```python
from build123d import *

# Parameters (mm, degrees)
BOSS_EXTRUDE1_DEPTH = 20
SKETCH2_W           = 700
SKETCH2_H           = 15
BOSS_EXTRUDE2_DEPTH = 20
SKETCH6_W           = 10
SKETCH6_H           = 10
BOSS_EXTRUDE3_DEPTH = 500
BOSS_EXTRUDE4_DEPTH = 5
SKETCH8_W           = 10
SKETCH8_H           = 10
BOSS_EXTRUDE5_DEPTH = 495
SKETCH4_W           = 700
SKETCH4_H           = 12.5
CUT_EXTRUDE2_DEPTH  = 5


with BuildPart() as part:
    # Sketch1 → Boss-Extrude1 (new body)
    with BuildSketch(Plane(origin=(0, 0, 0), x_dir=(1, 0, 0), z_dir=(0, 1, 0))):
        Polygon((0, 404.145188433), (-350, -202.072594216), (350, -202.072594216), align=None)
        Polygon((0, 381.051177665), (-330, -190.525588833), (330, -190.525588833), align=None, mode=Mode.SUBTRACT)
    extrude(amount=BOSS_EXTRUDE1_DEPTH)

    # Sketch2 → Boss-Extrude2 (add)
    with BuildSketch(Plane(origin=(0, 0, 0), x_dir=(1, 0, 0), z_dir=(0, 1, 0))):
        with Locations((0, -209.572594216)):
            Rectangle(SKETCH2_W, SKETCH2_H)
    extrude(amount=BOSS_EXTRUDE2_DEPTH)

    # Sketch6 → Boss-Extrude3 (add)
    with BuildSketch(Plane(origin=(0, 20, 0), x_dir=(1, 0, 0), z_dir=(0, 1, 0))):
        with Locations((40, -196.3)):
            Rectangle(SKETCH6_W, SKETCH6_H)
    extrude(amount=BOSS_EXTRUDE3_DEPTH)

    # Sketch7 → Boss-Extrude4 (add)
    with BuildSketch(Plane(origin=(0, 20, 0), x_dir=(1, 0, 0), z_dir=(0, 1, 0))):
        Polygon((62.94207364, 295.126318955), (-62.94207364, 295.126318955), (-95, 239.600361714), (95, 239.600361714), align=None)
    extrude(amount=BOSS_EXTRUDE4_DEPTH)

    # Sketch8 → Boss-Extrude5 (add)
    with BuildSketch(Plane(origin=(0, 25, 0), x_dir=(1, 0, 0), z_dir=(0, 1, 0))):
        with Locations((40, 250)):
            Rectangle(SKETCH8_W, SKETCH8_H)
    extrude(amount=BOSS_EXTRUDE5_DEPTH)

    # Sketch4 → Cut-Extrude2 (cut)
    with BuildSketch(Plane(origin=(0, 20, 0), x_dir=(1, 0, 0), z_dir=(0, 1, 0))):
        with Locations((0, -208.322594216)):
            Rectangle(SKETCH4_W, SKETCH4_H)
    extrude(amount=-CUT_EXTRUDE2_DEPTH, mode=Mode.SUBTRACT)


solid = part.part
```
The listing builds one solid part. Answer for the finished solid, in the listing's coordinates (mm). A direction names the side the tool comes from. Give positions to 0.01 mm unless a question says otherwise; leave off trailing zeros. Order: outer loops, then holes, each group sorted by start corner. A loop starts at its lowest first (then second) coordinate and runs counter-clockwise, first axis right, second up. Notation, with made-up numbers: (2.5, -6) -> (45.5, -6) arc R28 cw to (45.5, 22) -> close; hole circle Ø4 at (20, -4.75). An arc over 180 degrees is marked (long way). One line per item, written item: value.
1) Find section C-C, the plane x = 269. Determine the outline of the cut face in (y, z), plus the area to 3 significant figures.
Reported:
outline: (0, 61.78) -> (20, 61.78) -> (20, 84.87) -> (0, 84.87) -> close; (0, 190.53) -> (20, 190.53) -> (20, 202.07) -> (15, 202.07) -> (15, 214.57) -> (20, 214.57) -> (20, 217.07) -> (0, 217.07) -> close
area: 930 mm^2
2) A tool of negligible diameter and unlimited length cuts with its end or side. For faces 3 (the flat face through (-2, 0, 204)), 4 (the flat face through (-1, 20, -268)), from which of +Z, -Z, +X, -X, +Y, -Y can it reach the whole face along a straight path? Write none if from no direction.
Reported:
face 3: +Z, -Z, +X, -X, -Y
face 4: -Y
3) Determine the mould class of faces 1 (the flat face through (-5, 10, 190.526)), 2 (the flat face through (-14, 20, -358)) for opening direction X: pulls with the +X half, pulls with the -X half, needs draft (parallel to the pull), parting line crosses it, or undercut.
Reported:
face 1: undercut
face 2: needs draft
4) Find the intervals of material crossed by line 1 (Y direction, x = 15, z = -251.5), in increasing order.
Reported:
line 1: y = 20 to 25
5) Find section A-A, the plane y = 394. Determine the outline of the cut face in (x, z).
Reported:
outline: (35, -255) -> (45, -255) -> (45, -245) -> (35, -245) -> close; (35, 191.3) -> (45, 191.3) -> (45, 201.3) -> (35, 201.3) -> close
6) Flat-ended cylindrical pins translate along their axes: P1, Ø4, axis at x = 138.5, z = 205.5, coming from the +Y side; P2, Ø3, axis at x = 38.5, y = 356, coming from the -Z side; P3, Ø4, axis at x = -77.5, y = 18.5, coming from the -Z side. Find the tip coordinate at first contact, or state that the pin passes through.
Reported:
P1: stops at y = 15
P2: stops at z = -255
P3: stops at z = -273.38
7) Find section B-B, the plane z = 47.5. Determine the outline of the cut face in (x, y).
Reported:
outline: (-260.76, 0) -> (-247.42, 0) -> (-247.42, 20) -> (-260.76, 20) -> close; (247.42, 0) -> (260.76, 0) -> (260.76, 20) -> (247.42, 20) -> close
